Input: part model. Units: mm. Frame: model coordinates. A direction names the side the tool comes from. Coordinates: 2 decimals unless noted, no trailing zeros. Order: outer loops, then holes, each group sorted by start corner. A loop starts at its lowest first (then second) coordinate and runs counter-clockwise, first axis right, second up. Notation, with made-up numbers: (-7.75, 27) -> (2.25, 27) arc R16 cw to (2.25, 55) -> close; hole circle Ø5 at (77.5, 16). An arc over 180 degrees is marked (long way). Use one line per item in the form item = value. Start each with the question number.
1) Section query D-D on x = -19.5. Output: boundary loops of the cut face in (y, z).
2) Section query A-A on y = -25. Output: boundary loops of the cut face in (x, z), then the cut area to 3 significant figures.
3) Draft query along Z for faces 1 (the flat face through (-15, -21.9, 38.5)), 2 (the flat face through (0.49, 25.854, 10.14)), 3 (the flat face through (0, -30, 0)). Return one class per face: pulls with the +Z half, pulls with the -Z half, needs draft (parallel to the pull), parting line crosses it, or undercut.
4) Section query B-B on z = 10. Output: boundary loops of the cut face in (x, y).
5) Access query for faces 4 (the flat face through (16, -8, 30)), 5 (the flat face through (-25, -10, 37)), 6 (the flat face through (15, -21.9, 38.5)). Directions: +Z, -Z, +X, -X, +Y, -Y. A direction counts if a zero-diameter tool reaches every point of the face in a straight line with its end or side. Return the directions, or none.
6) Section query C-C on y = 24. Output: boundary loops of the cut face in (x, z).
7) Pin query (flat end, axial travel): pin 1 (16.5 mm diameter, centred on x = -27, z = 39.5, fed in from +Y); pin 2 (1.5 mm diameter, centred on x = -1, z = 56.5, fed in from -Y); pin 3 (12.5 mm diameter, centred on y = -25, z = 45, fed in from +X); pin 4 (2 mm diameter, centred on y = 22, z = 54, fed in from +X). Return the tip coordinate at first contact, or that it passes through.
8) Ray query, line 1 along Z through (x, y) = (26.5, -25); line 2 along X through (y, z) = (-29, 37); line 3 along Z through (x, y) = (17, 17.5). Return the intervals inside material, ascending.
from build123d import *

# Parameters (mm, degrees)
F1_DEPTH = 35
F2_R     = 7
F3_DEPTH = 20
F6_DEPTH = 30
F7_R     = 15
F8_DEPTH = 20


with BuildPart() as f1:
    # F0 (on Right) → F1 (new body, symmetric)
    with BuildSketch(Plane.YZ):
        Polygon((-40, 0), (-20, 0), (-31.5470053838, 20), (31.5470053838, 20), (20, 0), (40, 0), (40, 30), (-40, 30), align=None)
    extrude(amount=F1_DEPTH, both=True)

    # F2 (on face) → F3 (join)
    with BuildSketch(Plane.YZ.offset(35)):
        with BuildLine():
            Line((-10, 30), (-10, 45))
            ThreePointArc((-10, 45), (-25, 60), (-40, 45))
            Line((-40, 45), (-40, 30))
            Line((-40, 30), (-10, 30))
        make_face()
        with Locations((-25, 45)):
            Circle(F2_R, mode=Mode.SUBTRACT)
    extrude(amount=-F3_DEPTH)

    # F4: F1 across plane


with BuildPart() as f1_1:
    add(f1.part)
    add(f1.part.mirror(Plane.YZ))

    # F5 (on face) → F6 (join)
    with BuildSketch(Plane.XY.offset(30)):
        with BuildLine():
            ThreePointArc((3.22e-08, 40), (-17.6776695411, -2.6776695183), (25, 15))
            ThreePointArc((25, 15), (17.6776695411, 32.6776695183), (3.22e-08, 40))
        make_face()
    extrude(amount=F6_DEPTH)

    # F7 (on face) → F8 (join)
    with BuildSketch(Plane.XY.offset(60)):
        with Locations((0, 15)):
            Circle(F7_R)
    extrude(amount=F8_DEPTH)


solid = f1_1.part
Answers below:
q1.outline = (-40, 0) -> (-20, 0) -> (-31.55, 20) -> (31.55, 20) -> (20, 0) -> (40, 0) -> (40, 30) -> (30.64, 30) -> (30.64, 60) -> (-0.64, 60) -> (-0.64, 30) -> (-10, 30) -> (-10, 45) arc R15 ccw to (-40, 45) -> close; hole circle Ø14 at (-25, 45)
q2.outline = (-35, 0) -> (35, 0) -> (35, 8.66) -> (-35, 8.66) -> close; (-35, 20) -> (35, 20) -> (35, 38) -> (15, 38) -> (15, 30) -> (-15, 30) -> (-15, 38) -> (-35, 38) -> close; (-35, 52) -> (-15, 52) -> (-15, 60) -> (-35, 60) -> close; (15, 52) -> (35, 52) -> (35, 60) -> (15, 60) -> close
q2.area = 1,950 mm^2
q3.face_1 = needs draft
q3.face_2 = undercut
q3.face_3 = pulls with the -Z half
q4.outline = (-35, -40) -> (35, -40) -> (35, -25.77) -> (-35, -25.77) -> close; (-35, 25.77) -> (35, 25.77) -> (35, 40) -> (-35, 40) -> close
q5.face_4 = +Z
q5.face_5 = +Z, -X
q5.face_6 = +Z, -Y
q6.outline = (-35, 0) -> (35, 0) -> (35, 6.93) -> (-35, 6.93) -> close; (-35, 20) -> (35, 20) -> (35, 30) -> (23.32, 30) -> (23.32, 60) -> (12, 60) -> (12, 80) -> (-12, 80) -> (-12, 60) -> (-23.32, 60) -> (-23.32, 30) -> (-35, 30) -> close
q7.pin_1 = 31.54
q7.pin_2 = -10
q7.pin_3 = through
q7.pin_4 = 24.27
q8.line_1 = 0 to 8.66, 20 to 38, 52 to 60
q8.line_2 = -35 to -15, 15 to 35
q8.line_3 = 20 to 60
